Work out the finished part from the listing and answer in its coordinate system (mm). Face numbers are marked on the shaded views. Coordinates: 2 decimals unless noted, no trailing zeros. Write each loop counter-clockwise with the first axis right and the second up, starting at its lowest first coordinate (ties: lowest second). Pieces come first, ordered by that corner, then holes. Notation, with made-up numbers: (8.5, 65) - (62.5, 65) arc R27 cw to (62.5, 83) - close; hole circle Ø4 at (85.25, 34.25). An arc over 180 degrees is marked (long way). Use a Markdown table: item, result. Add a question column.
(1) The part is cut by section B-B, the plane z = 0. Give the vertices of the cut face in (x, y) (3 decimals), then the cut area to 3 significant figures.
(2) Find the intervals of material crossed by line 1 (Z direction, x = 0, y = -4.5) (1 decimal); line 2 (X direction, y = -2, z = 0) (3 decimals); line 3 (X direction, y = -1.5, z = -21), in increasing order. Write a range as from..to.
(3) For a pull along X with two mould halves and no side action, classify the marked faces 1, 2, 3 and 4 as released by +X, released by -X, zero draft, split by the parting line, or undercut.
(4) Given pin 1 Ø3 at (y, z) = (-4.5, 23) entering from -X; pin 2 Ø4 at (x, y) = (18.5, -1.5) entering from -Z; pin 3 Ø3 at (y, z) = (-3, -3.5) entering from +X, each flat-ended and moving along its own axis, determine where each tip first touches the part or whether it passes through.
(5) The part is cut by section A-A, the plane x = 0. State how many separate pieces and enclosed holes the cut face has, then the cut area to 3 significant figures.
from build123d import *

# Parameters (mm, degrees)
SKETCH1_W               = 20.865197439
SKETCH1_H               = 9.525
SKETCH2_R               = 4.7625
SKETCH2_R_2             = 15.875
CUT_EXTRUDE1_DEPTH      = 16.875
CUT_EXTRUDE1_DEPTH_BACK = 1
FILLET1_R               = 6.35


with BuildPart() as part:
    # Sketch1 → Revolve1 (revolve)
    with BuildSketch(Plane.XY):
        Polygon((31.839802561, 6.35), (26.759802561, 1.27), (26.759802561, 0), (47.625, 0), (47.625, 6.35), align=None)
        with Locations((37.192401281, -4.7625)):
            Rectangle(SKETCH1_W, SKETCH1_H)
    revolve(axis=Axis((0, 0, 0), (0, 1, 0)))

    # Sketch2 → Cut-Extrude1 (cut, two sides)
    with BuildSketch(Plane(origin=(0, 6.35, 0), x_dir=(-1, 0, 0), z_dir=(0, -1, 0))) as cut_extrude1_sk:
        with Locations((0, 38.1)):
            Circle(SKETCH2_R)
        with Locations((32.995567884, 19.05)):
            Circle(SKETCH2_R)
        with Locations((32.995567884, -19.05)):
            Circle(SKETCH2_R)
        with Locations((0, -38.1)):
            Circle(SKETCH2_R)
        with Locations((-32.995567884, -19.05)):
            Circle(SKETCH2_R)
        with Locations((-32.995567884, 19.05)):
            Circle(SKETCH2_R)
        with Locations((50.8, 0)):
            Circle(SKETCH2_R_2)
        with Locations((25.4, -43.994090512)):
            Circle(SKETCH2_R_2)
        with Locations((-25.4, -43.994090512)):
            Circle(SKETCH2_R_2)
        with Locations((-50.8, 0)):
            Circle(SKETCH2_R_2)
        with Locations((-25.4, 43.994090512)):
            Circle(SKETCH2_R_2)
        with Locations((25.4, 43.994090512)):
            Circle(SKETCH2_R_2)
    extrude(amount=CUT_EXTRUDE1_DEPTH, mode=Mode.SUBTRACT)
    extrude(cut_extrude1_sk.sketch, amount=-CUT_EXTRUDE1_DEPTH_BACK, mode=Mode.SUBTRACT)

    # Fillet1
    fillet1_edges = [part.edges().sort_by_distance(p)[0] for p in [
        (-35.500453462, -1.5875, 31.746786121),
        (-9.743296538, -1.5875, 46.617687604),
        (-45.24375, -1.5875, -14.870901484),
        (-45.24375, -1.5875, 14.870901484),
        (9.743296538, -1.5875, 46.617687604),
        (35.500453462, -1.5875, 31.746786121),
        (45.24375, -1.5875, 14.870901484),
        (45.24375, -1.5875, -14.870901484),
        (35.500453462, -1.5875, -31.746786121),
        (9.743296538, -1.5875, -46.617687604),
        (-9.743296538, -1.5875, -46.617687604),
        (-35.500453462, -1.5875, -31.746786121),
    ]]
    fillet(fillet1_edges, radius=FILLET1_R)


solid = part.part
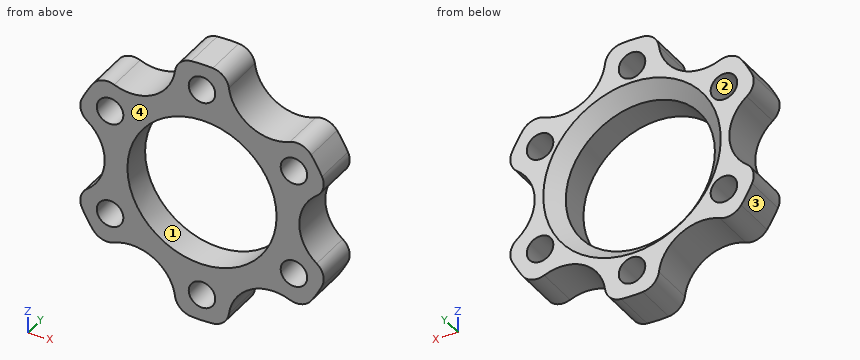
Model answer:
| question | item | result |
|---|---|---|
| 1 | outline | (-34.925, -9.525) - (-26.76, -9.525) - (-26.76, 1.27) - (-31.84, 6.35) - (-34.925, 6.35) - close; (26.76, -9.525) - (34.925, -9.525) - (34.925, 6.35) - (31.84, 6.35) - (26.76, 1.27) - close |
| 1 | area | 233 mm^2 |
| 2 | line 1 | -47.6..-42.9, -33.3..-26.8, 26.8..33.3, 42.9..47.6 |
| 2 | line 2 | -34.925..-26.76, 26.76..34.925 |
| 2 | line 3 | -42.75..-37.34, -28.65..-16.59, 16.59..28.65, 37.34..42.75 |
| 3 | face 1 | undercut |
| 3 | face 2 | undercut |
| 3 | face 3 | released by -X |
| 3 | face 4 | zero draft |
| 4 | pin 1 | x = -42.5 |
| 4 | pin 2 | z = -30.85 |
| 4 | pin 3 | x = 35.73 |
| 5 | separate pieces | 4 |
| 5 | enclosed holes | 0 |
| 5 | area | 334 mm^2 |
